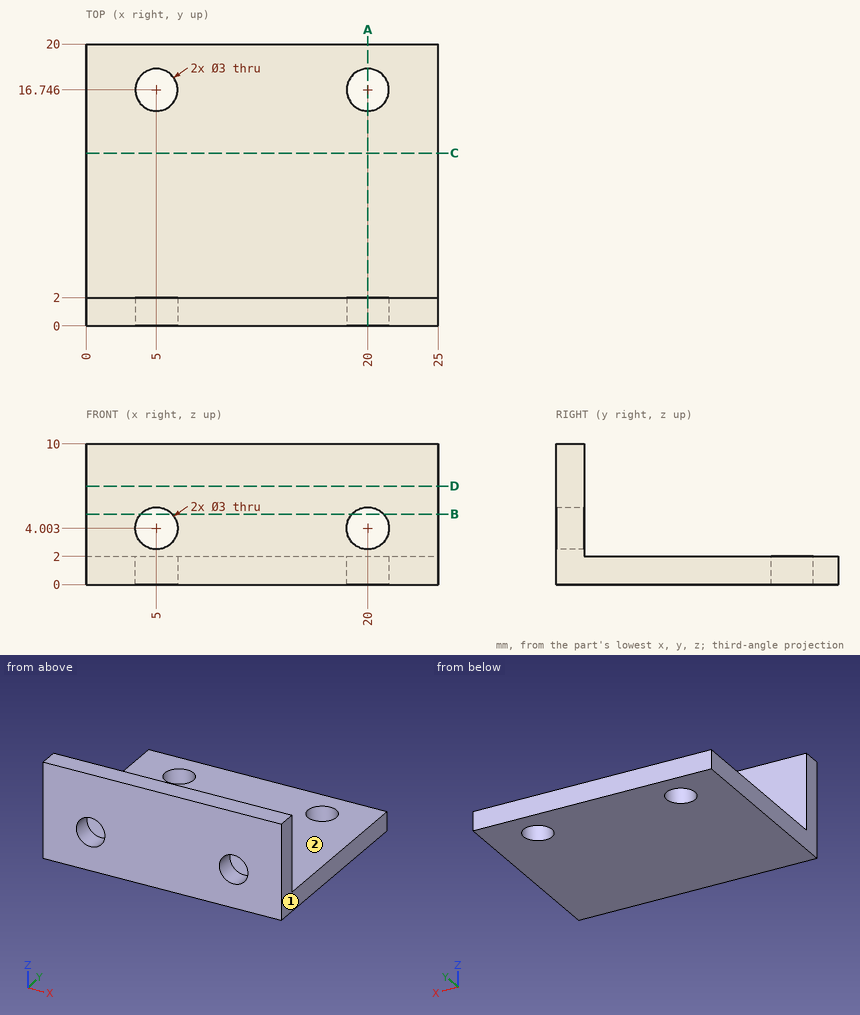
For this review, use the dimensioned drawing (mm, ordinates from the lowest corner) and the shaded views. A direction names the side the tool comes from. Give positions to 0.01 mm unless a question says otherwise; leave off trailing zeros. Order: outer loops, then holes, each group sorted by start corner. A loop starts at its lowest first (then second) coordinate and runs counter-clockwise, first axis right, second up.
1) Wall thickness on line 1 (Y direction, x = 5, z = 1.1) (1 decimal); line 2 (Z direction, x = 11.5, y = 2.75): over which ranges is each line inside the solid? List them lowest first.
2) For the marked faces 1 and 2, list the 3-axis set-ups (+Z, -Z, +X, -X, +Y, -Y) from which the entire face can be reached by the end or side of a thin tool; tool diameter is ignored.
3) Insertion check: pin 1 (2 mm diameter, centred on y = 6, z = 3.5, fed in from -X); pin 2 (10 mm diameter, centred on x = 6, y = 12, fed in from +Z). Each pin has a flat end and moves straight along its axis. Give the tip position at first contact, or say it passes through.
4) Take a section at A-A (x = 20). Give the boundary of the cut face in (y, z) (1 decimal).
5) Take a section at C-C (y = 12.25). Give the boundary of the cut face in (x, z).
6) Take a section at B-B (z = 5). Give the boundary of the cut face in (x, y).
Derived:
1. line 1: y = 0 to 15.2, 18.2 to 20
1. line 2: z = 0 to 2
2. face 1: +Z, -Z, +X, +Y, -Y
2. face 2: +Z, +X, -X, +Y
3. pin 1: passes through
3. pin 2: stops at z = 2
4. outline: (0, 0) - (15.2, 0) - (15.2, 2) - (2, 2) - (2, 2.5) - (0, 2.5) - close; (0, 5.5) - (2, 5.5) - (2, 10) - (0, 10) - close; (18.2, 0) - (20, 0) - (20, 2) - (18.2, 2) - close
5. outline: (0, 0) - (25, 0) - (25, 2) - (0, 2) - close
6. outline: (0, 0) - (3.88, 0) - (3.88, 2) - (0, 2) - close; (6.12, 0) - (18.88, 0) - (18.88, 2) - (6.12, 2) - close; (21.12, 0) - (25, 0) - (25, 2) - (21.12, 2) - close
